from build123d import *

# Parameters (mm, degrees)
EXTRUDE_2_DEPTH = 1
EXTRUDE_3_DEPTH = 1


with BuildPart() as part:
    # 草图1 → 凸台-拉伸2 (new body)
    with BuildSketch(Plane.XY):
        Polygon((-57.86, -80), (-57.86, 70), (-56.46, 70), (-56.46, -80), (-34.28, -80), (-29.28, -80), (-29.28, 70), (-27.88, 70), (-27.88, -80), (-5.7, -80), (-0.7, -80), (-0.7, 70), (0.7, 70), (0.7, -80), (22.88, -80), (27.88, -80), (27.88, 70), (29.28, 70), (29.28, -80), (51.46, -80), (56.46, -80), (56.46, 70), (57.86, 70), (57.86, -80), (80, -80), (80, 80), (-80, 80), (-80, -80), (-62.86, -80), align=None)
    extrude(amount=EXTRUDE_2_DEPTH)

    # 草图2 → 凸台-拉伸3 (add)
    with BuildSketch(Plane(origin=(0, 0, 0), x_dir=(-1, 0, 0), z_dir=(0, 0, -1))):
        Polygon((-80, -70), (-77.5, -70), (-77.5, -67.5), (-72.5, -67.5), (-72.5, -70), (-70, -70), (-70, 70), (72.5, 70), (72.5, 72.5), (77.5, 72.5), (77.5, 70), (80, 70), (80, 80), (-80, 80), align=None)
    extrude(amount=EXTRUDE_3_DEPTH)


solid = part.part
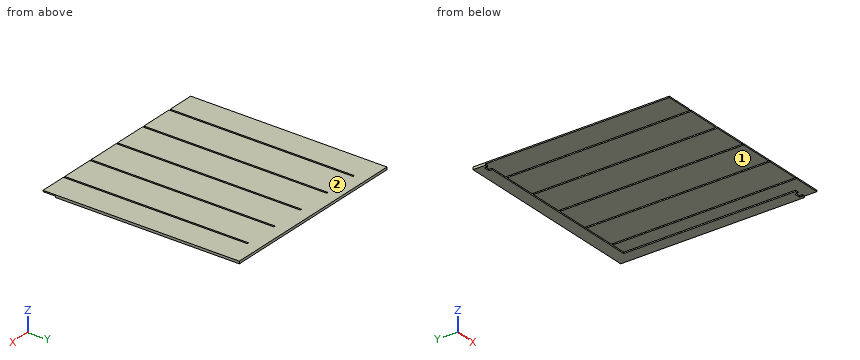
Could you check a few things on this model? Use its own coordinates, in mm. Face numbers are marked on the shaded views. A direction names the side the tool comes from. Coordinates: 2 decimals unless noted, no trailing zeros. Order: outer loops, then holes, each group sorted by start corner. A loop starts at its lowest first (then second) coordinate and runs counter-clockwise, first axis right, second up. Notation, with made-up numbers: (-10, 35) -> (-4, 35) arc R13 ccw to (-4, 60) -> close; hole circle Ø11 at (-6.75, 10.5). An arc over 180 degrees is marked (long way). One line per question, with ' | ' between items.
Q1. Imagine slicing it at B-B on z = -0.4. Please give me the cut outline in (x, y), and give its area (4 significant figures).
Return value:
outline: (-80, 70) -> (-77.5, 70) -> (-77.5, 72.5) -> (-72.5, 72.5) -> (-72.5, 70) -> (70, 70) -> (70, -70) -> (72.5, -70) -> (72.5, -67.5) -> (77.5, -67.5) -> (77.5, -70) -> (80, -70) -> (80, 80) -> (-80, 80) -> close | area: 2,975 mm²
Q2. I'm going to push flat-ended pins straight in: P1, Ø11, axis at x = -71, y = -4, coming from the -Z side; P2, Ø0.8, axis at x = 74, z = -0.5, coming from the -Y side; P3, Ø0.8, axis at x = -78.5, z = -0.5, coming from the -Y side. Where does each tip first touch, or does it pass through?
Return value:
P1: z = 0 | P2: y = -67.5 | P3: y = 70
Q3. On a 3-axis mill with a long thin cutter (end or side, diameter ignored), from which of +Z, -Z, +X, -X, +Y, -Y can I reach the whole of each face in a straight line? I mean the marked faces 1 and 2. Say none if no direction works.
Return value:
face 1: -Z, -X, -Y | face 2: +Z, +X, -X, +Y, -Y
Q4. Imagine slicing it at A-A on y = -6. Please give me the cut outline in (x, z), and give its area (3 significant figures).
Return value:
outline: (-80, 0) -> (-57.86, 0) -> (-57.86, 1) -> (-80, 1) -> close; (-56.46, 0) -> (-29.28, 0) -> (-29.28, 1) -> (-56.46, 1) -> close; (-27.88, 0) -> (-0.7, 0) -> (-0.7, 1) -> (-27.88, 1) -> close; (0.7, 0) -> (27.88, 0) -> (27.88, 1) -> (0.7, 1) -> close; (29.28, 0) -> (56.46, 0) -> (56.46, 1) -> (29.28, 1) -> close; (57.86, 0) -> (70, 0) -> (70, -1) -> (80, -1) -> (80, 1) -> (57.86, 1) -> close | area: 163 mm²
Q5. If I drill on L1, parallel to X at y = 63, z = 0.1; L2, parallel to Z at x = -64, y = -55.5; L3, parallel to Y at x = -45.5, z = -0.75, over which ranges is the centre line in solid material (lowest first)?
Return value:
L1: -80 to -57.86, -56.46 to -29.28, -27.88 to -0.7, 0.7 to 27.88, 29.28 to 56.46, 57.86 to 80 | L2: 0 to 1 | L3: 70 to 80
Q6. Imagine slicing it at C-C on x = -5. Please give me the cut outline in (y, z).
Return value:
outline: (-80, 0) -> (70, 0) -> (70, -1) -> (80, -1) -> (80, 1) -> (-80, 1) -> close
